Work out the finished part from the listing and answer in its coordinate system (mm). A direction names the side the tool comes from. Coordinates: 2 decimals unless noted, no trailing zeros. Write each loop counter-clockwise with the first axis right and the second up, starting at its lowest first coordinate (ties: lowest second). Pieces come first, ordered by that corner, then holes. Notation, with made-up numbers: (60.25, -25) - (67.25, -25) arc R22 cw to (67.25, -16) - close; hole circle Ø7 at (74.25, 34.5). An arc over 180 degrees is marked (long way). Use a Markdown table: item, result. Add a question column.
(1) Given pin 1 Ø0.5 at (x, y) = (10.5, 0.5) entering from -Z, flat-ended and moving along its own axis, determine where the tip first touches the part or whether it passes through.
(2) The part is cut by section D-D, the plane x = 5. Give the vertices of the cut face in (y, z).
(3) Find the intervals of material crossed by line 1 (Z direction, x = 10, y = 0.95); line 2 (Z direction, x = 11.5, y = 1.2); line 3 (X direction, y = 1.2, z = 21.7), in increasing order. Write a range as from..to.
(4) The part is cut by section C-C, the plane y = 0.3. Give the vertices of the cut face in (x, z), then the cut area to 3 significant figures.
(5) The part is cut by section A-A, the plane x = 10. Give the vertices of the cut face in (y, z).
(6) A tool of negligible diameter and unlimited length cuts with its end or side. For faces 1 (the face through (10, 1, 21)), 2 (the face through (3, 1, -26)), 3 (the face through (-11.504, 0.811, 13.821)), from which of +Z, -Z, +X, -X, +Y, -Y can it reach the whole face along a straight path? Write none if from no direction.
(7) The part is cut by section B-B, the plane z = -22.3. Give the vertices of the cut face in (x, y).
(8) For a pull along X with two mould halves and no side action, classify faces 4 (the face through (14, 1, 0)), 5 (the face through (-4.301, 0.811, 20.604)), 6 (the face through (-1.67, 0.81, -23.59)), 7 (the face through (11, 1, -21)) as released by +X, released by -X, zero draft, split by the parting line, or undercut.
Autodesk Inventor part; units mm, degrees
ref_plane "YZ Plane" through (0, 0, 0) normal (1, 0, 0) x (0, 1, 0)
ref_plane "XZ Plane" through (0, 0, 0) normal (0, 1, 0) x (-1, 0, 0)
ref_plane "XY Plane" through (0, 0, 0) normal (0, 0, 1) x (1, 0, 0)
sketch "Esquisse1" plane through (0, 0, 0) normal (0, 1, 0) x (-1, 0, 0)
  line L0 (14, -28) -> (-14, -28)
  line L1 (-14, -28) -> (-14, 28)
  line L2 (-14, 28) -> (14, 28)
  line L3 (14, 28) -> (14, -28)
  point P0 (0, 0)
  dimension "d0" = 28
  dimension "d1" = 56
  dimension "d2" = 28
  dimension "d3" = 14
extrude "Extrusion1" add sketch "Esquisse1" along normal blind 1.6
fillet "Congé1" radius 15 2 edges at (-14, 0.8, -28) (-14, 0.8, 28)
sketch "Esquisse2" plane through (0, 1.6, 0) normal (0, 1, 0) x (1, 0, 0)
  circle A0 centre (7, 25) radius 4
  circle A1 centre (7, -25) radius 4
  line L0 (1, -28) -> (14, -28)
  line L1 (3, 25) -> (3, 28)
  line L2 (14, 28) -> (1, 28)
  line L3 (4.3542, 28) -> (3, 28)
  line L4 (9.6458, 28) -> (14, 28)
  line L5 (14, 28) -> (14, 21)
  line L6 (14, -28) -> (14, 28)
  line L7 (14, 21) -> (7, 21)
  line L8 (7, -21) -> (14, -21)
  line L9 (14, -21) -> (14, -28)
  line L10 (14, -28) -> (9.6458, -28)
  line L11 (3, -25) -> (3, -28)
  line L12 (3, -28) -> (4.3542, -28)
  point P0 (0, 0)
  dimension "d7" = 8
  dimension "d8" = 7
  dimension "d9" = 7
  dimension "d10" = 25
  dimension "d11" = 25
extrude "Extrusion3" cut sketch "Esquisse2" against normal through all contours A0 L2 | A0 L2 L5 L7 | L6 L0 A1 L8 | A0 L1 L2 | A1 L0 | A1 L0 L11 picked at (8.3035, 24.6872) picked at (8.2117, -25.5325)
sketch "Esquisse3" plane through (0, 1.6, 0) normal (0, 1, 0) x (1, 0, 0)
  circle A0 centre (-5, -21.7) radius 1.3
  line L0 (-14, 13) -> (-14, -13)
  circle A1 centre (-1.5, 22.3) radius 1.3
  circle A2 centre (10, -15.2) radius 1.3
  point P0 (0, 0)
  dimension "d21" = 2.6
  dimension "d23" = 9
  dimension "d30" = 21.7
  dimension "d31" = 2.6
  dimension "d32" = 12.5
  dimension "d33" = 9.3
  dimension "d34" = 2.6
  dimension "d35" = 6.5
  dimension "d36" = 15
extrude "Extrusion4" cut sketch "Esquisse3" against normal through all
sketch "Esquisse4" plane through (0, 1.6, 0) normal (0, 1, 0) x (1, 0, 0)
  circle A0 centre (-14, -13.969) radius 2.5
  line L0 (14, -21) -> (14, 21)
  line L1 (7, -21) -> (14, -21)
  point P0 (0, 0)
  dimension "d37" = 5
  dimension "d38" = 28
  dimension "d39" = 7.031
extrude "Extrusion5" cut sketch "Esquisse4" against normal through all
equation "\"d31\" = d21"
equation "\"d34\" = d21"
properties part number "PCB Gauche" material "Nylon, disulfure de molybdène"
Model answer:
| question | item | result |
|---|---|---|
| 1 | pin 1 | z = -21 |
| 2 | outline | (0, -21.54) - (1.6, -21.54) - (1.6, 21.54) - (0, 21.54) - close |
| 3 | line 1 | -21..13.9, 16.5..21 |
| 3 | line 2 | -21..21 |
| 3 | line 3 | -11.22..-6.3, -3.7..4.74 |
| 4 | outline | (-14, -13) arc R15 ccw to (1, -28) - (3, -28) - (3, -25) arc R4 cw to (7, -21) - (14, -21) - (14, 21) - (7, 21) arc R4 cw to (3, 25) - (3, 28) - (1, 28) arc R15 ccw to (-13.6, 16.44) arc R2.5 cw to (-14, 11.47) - close; hole circle Ø2.6 at (-5, 21.7); hole circle Ø2.6 at (-1.5, -22.3); hole circle Ø2.6 at (10, 15.2) |
| 4 | area | 1,300 mm^2 |
| 5 | outline | (0, -21) - (1.6, -21) - (1.6, 13.9) - (0, 13.9) - close; (0, 16.5) - (1.6, 16.5) - (1.6, 21) - (0, 21) - close |
| 6 | face 1 | +Z, +X, +Y, -Y |
| 6 | face 2 | -Z, +X, +Y, -Y |
| 6 | face 3 | -X, +Y, -Y |
| 7 | outline | (-10.77, 0) - (-2.8, 0) - (-2.8, 1.6) - (-10.77, 1.6) - close; (-0.2, 0) - (4.05, 0) - (4.05, 1.6) - (-0.2, 1.6) - close |
| 8 | face 4 | released by +X |
| 8 | face 5 | undercut |
| 8 | face 6 | undercut |
| 8 | face 7 | zero draft |
